```python
from build123d import *

# Parameters (mm, degrees)
F1_DEPTH = 3
F2_W     = 7
F2_H     = 7
F4_W     = 7
F4_H     = 7
F6_W     = 7
F6_H     = 22
F7_DEPTH = 3
F8_R     = 3


with BuildPart() as f1:
    # F0 (on Front) → F1 (new body)
    with BuildSketch(Plane.XZ):
        Polygon((-13, 49), (-20, 49), (-20, 0), (0, 0), (0, 7), (-13, 7), align=None)
    extrude(amount=F1_DEPTH)

    # F2 (on face) → F5 section 0
    with BuildSketch(Plane(origin=(0, 0, 0), x_dir=(-1, 0, 0), z_dir=(0, 1, 0))):
        with Locations((16.5, 45.5)):
            Rectangle(F2_W, F2_H)
    # F4 (on offset) → F5 section 1
    with BuildSketch(Plane(origin=(0, 40, 0), x_dir=(-1, 0, 0), z_dir=(0, 1, 0))):
        with Locations((30.5, 45.5)):
            Rectangle(F4_W, F4_H)
    loft()

    # F6 (on face) → F7 (join)
    with BuildSketch(Plane(origin=(0, 40, 0), x_dir=(-1, 0, 0), z_dir=(0, 1, 0))):
        with Locations((30.5, 38)):
            Rectangle(F6_W, F6_H)
    extrude(amount=F7_DEPTH)

    # F8
    f8_edges = [f1.edges().sort_by_distance(p)[0] for p in [
        (-13, -1.5, 7),
        (-20, -1.5, 0),
        (-16.5, -3, 49),
        (-16.5, 0, 42),
        (-30.5, 40, 42),
        (-30.5, 43, 49),
    ]]
    fillet(f8_edges, radius=F8_R)

    # F9: F1 across plane


with BuildPart() as f1_1:
    add(f1.part)
    add(f1.part.mirror(Plane.YZ))


solid = f1_1.part
```
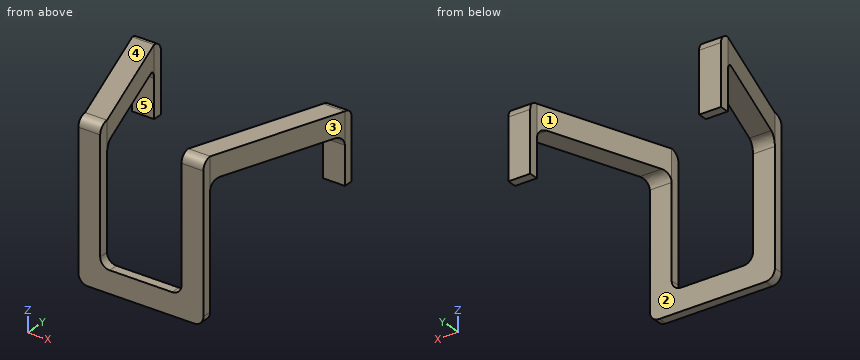
Check sheet for the modelled part. Datum: model origin and axes. Units: mm. Face numbers are marked on the shaded views. A direction names the side the tool comes from. Round coordinates to 2 decimals unless told otherwise and drop trailing zeros. Loops run counter-clockwise (first coordinate to the right, second up) from the corner with the lowest first, then second, coordinate; pieces in that order, holes last. Notation, with made-up numbers: M 87.5,5.25 L 116.5,5.25 A35 ccw 116.5,37.25 Z; hole C 68,8.25 d5. An arc over 180 degrees is marked long. Answer as a JSON object with one key per item and string values.
1. Section check D-D (z = 40.5). State how many separate pieces and enclosed holes the cut face has, plus the area to 3 significant figures.
Reply:
{"separate pieces": "4", "enclosed holes": "0", "area": "95.3 mm²"}
2. Access from +Z, -Z, +X, -X, +Y, -Y to the whole of each face (thin tool, end or side, straight path). Record for the marked faces 4 and 5.
Reply:
{"face 4": "+Z, +X, -X, +Y, -Y", "face 5": "-Z, +X, -X, -Y"}
3. Gauge pin test, flat ends, axial feed: P1, Ø1.5, axis at x = -29, y = 41, coming from the -Z side; P2, Ø5.5, axis at x = 29.5, z = 35, coming from the -Y side; P3, Ø1.5, axis at y = -1.5, z = 28, coming from the +X side. Record the tip position at first contact, or that the pin passes through.
Reply:
{"P1": "stops at z = 27", "P2": "stops at y = 40", "P3": "stops at x = 20"}
4. Scan lines: line 1 (X direction, y = -1, z = 18); line 2 (X direction, y = 2, z = 44.5); line 3 (Z direction, x = -26.5, y = 37). Record each from-to range of solid material in increasing order.
Reply:
{"line 1": "x = -20 to -13, 13 to 20", "line 2": "x = -20.7 to -13.7, 13.7 to 20.7", "line 3": "z = 42 to 49"}
5. Section check C-C (x = -3). Record the boundary of the cut face in (y, z).
Reply:
{"outline": "M -3,0 L 0,0 L 0,7 L -3,7 Z"}
6. Section check B-B (z = 34). Record the boundary of the cut face in (x, y).
Reply:
{"outline": "M -34,40 L -27,40 L -27,43 L -34,43 Z; M -20,-3 L -13,-3 L -13,0 L -20,0 Z; M 13,-3 L 20,-3 L 20,0 L 13,0 Z; M 27,40 L 34,40 L 34,43 L 27,43 Z"}
7. Mould release check, pull along X, two halves, no side actions. Record for the marked faces 1, 2 and 3: pulls with the +X half, pulls with the -X half, needs draft (parallel to the pull), parting line crosses it, or undercut.
Reply:
{"face 1": "undercut", "face 2": "needs draft", "face 3": "pulls with the +X half"}
8. Section check A-A (z = 11). Record the boundary of the cut face in (x, y).
Reply:
{"outline": "M -20,-3 L -13,-3 L -13,0 L -20,0 Z; M 13,-3 L 20,-3 L 20,0 L 13,0 Z"}
